Answer from the drawing. Dimensions are ordinates in mm from the lowest x, y and z of the part. Round coordinates to 2 decimals unless told otherwise and drop trailing zeros. Loops run counter-clockwise (first coordinate to the right, second up) from the corner with the lowest first, then second, coordinate; pieces in that order, holes last.
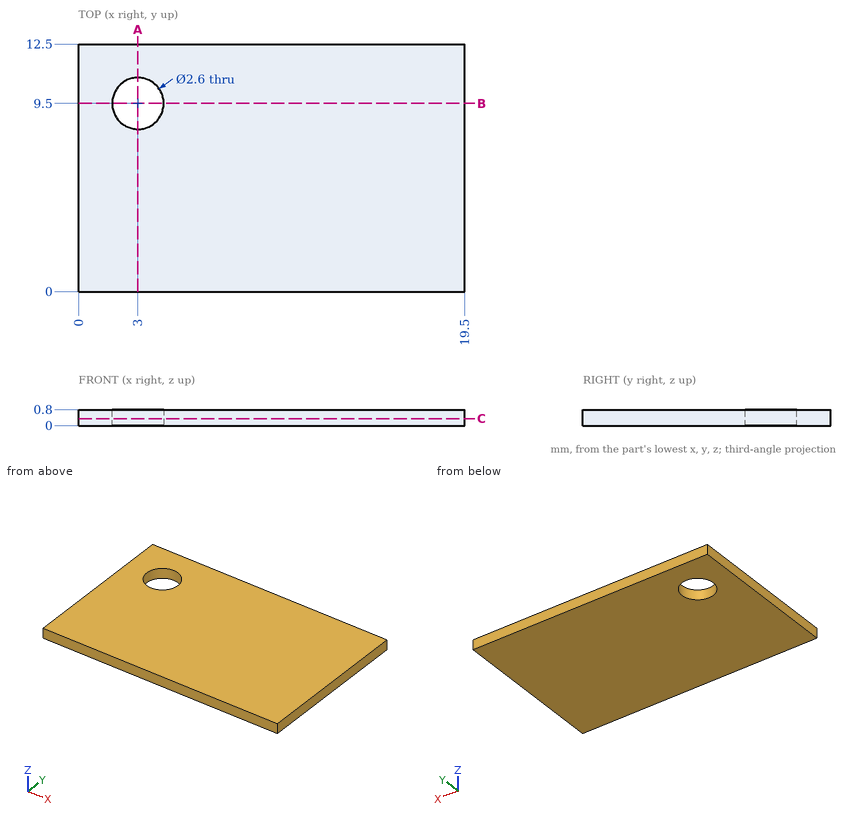
Item 1: Straight lines are drawn through the part: line 1 (Y direction, x = 3, z = 0.3); line 2 (X direction, y = 9.25, z = 0.25). For each, find the intervals that lie inside material, in ascending order.
Item 2: Section B-B, the plane y = 9.5 is taken. Give the vertices of the cut face in (x, z), plus the area to 3 significant figures.
Item 3: Section A-A, the plane x = 3 is taken. Give the vertices of the cut face in (y, z).
Item 4: Section C-C, the plane z = 0.35 is taken. Give the vertices of the cut face in (x, y).
Answer below:
1. line 1: y = 0 to 8.2, 10.8 to 12.5
1. line 2: x = 0 to 1.72, 4.28 to 19.5
2. outline: (0, 0) - (1.7, 0) - (1.7, 0.8) - (0, 0.8) - close; (4.3, 0) - (19.5, 0) - (19.5, 0.8) - (4.3, 0.8) - close
2. area: 13.5 mm2
3. outline: (0, 0) - (8.2, 0) - (8.2, 0.8) - (0, 0.8) - close; (10.8, 0) - (12.5, 0) - (12.5, 0.8) - (10.8, 0.8) - close
4. outline: (0, 0) - (19.5, 0) - (19.5, 12.5) - (0, 12.5) - close; hole circle Ø2.6 at (3, 9.5)
